For this review, take the finished solid that the model builds, in its own axes (mm). Face numbers are marked on the shaded views. A direction names the side the tool comes from. Round coordinates to 2 decimals unless told otherwise and drop trailing zeros. Order: outer loops, then holes, each group sorted by start corner. A loop starts at its lowest first (then second) coordinate and runs counter-clockwise, first axis right, second up.
from build123d import *

# Parameters (mm, degrees)
F0_W      = 143.89868
F0_H      = 139.25679
F1_DEPTH  = 152.4
F2_W      = 25.4
F2_H      = 25.4
F2_W_2    = 35.657714
F2_H_2    = 78.153904
F3_DEPTH  = 142.24
F4_W      = 129.092633
F4_H      = 89.404348
F5_DEPTH  = 50.8
F6_W      = 134.386524
F6_H      = 100.197379
F7_DEPTH  = 50.8
F8_W      = 129.092633
F8_H      = 8.289584
F9_DEPTH  = 50.8
F10_W     = 25.4
F10_H     = 25.4
F11_DEPTH = 25.4
F12_W     = 25.4
F12_H     = 25.4
F13_DEPTH = 50.8
F14_W     = 25.399997
F14_H     = 25.4
F14_W_2   = 25.4
F15_DEPTH = 25.4


with BuildPart() as f1:
    # F0 (on Front) → F1 (new body)
    with BuildSketch(Plane.XZ):
        Rectangle(F0_W, F0_H)
    extrude(amount=F1_DEPTH)

    # F2 (on face) → F3 (cut)
    with BuildSketch(Plane.XZ.offset(152.4)):
        with Locations((-40.786578, 12.7)):
            Rectangle(F2_W, F2_H)
        with Locations((40.542332, 12.7)):
            Rectangle(F2_W, F2_H)
        with Locations((0, -15.630781)):
            Rectangle(F2_W_2, F2_H_2)
    extrude(amount=-F3_DEPTH, mode=Mode.SUBTRACT)

    # F4 (on face) → F5 (cut)
    with BuildSketch(Plane.YZ.offset(-17.828857)):
        with Locations((-79.17279, -1.715975)):
            Rectangle(F4_W, F4_H)
    extrude(amount=-F5_DEPTH, mode=Mode.SUBTRACT)

    # F6 (on face) → F7 (cut)
    with BuildSketch(Plane(origin=(17.828857, 0, 0), x_dir=(0, -1, 0), z_dir=(-1, 0, 0))):
        with Locations((77.042945, -4.609043)):
            Rectangle(F6_W, F6_H)
    extrude(amount=-F7_DEPTH, mode=Mode.SUBTRACT)

    # F8 (on face) → F9 (cut)
    with BuildSketch(Plane.YZ.offset(-17.828857)):
        with Locations((-79.17279, -50.562941)):
            Rectangle(F8_W, F8_H)
    extrude(amount=-F9_DEPTH, mode=Mode.SUBTRACT)

    # F10 (on face) → F11 (cut)
    with BuildSketch(Plane.YZ.offset(71.94934)):
        with Locations((-115.364381, 20.59305)):
            Rectangle(F10_W, F10_H)
        with Locations((-39.158143, 20.59305)):
            Rectangle(F10_W, F10_H)
    extrude(amount=-F11_DEPTH, mode=Mode.SUBTRACT)

    # F12 (on face) → F13 (cut)
    with BuildSketch(Plane(origin=(-71.94934, 0, 0), x_dir=(0, -1, 0), z_dir=(-1, 0, 0))):
        with Locations((46.475742, 16.083911)):
            Rectangle(F12_W, F12_H)
        with Locations((105.357133, 16.083911)):
            Rectangle(F12_W, F12_H)
    extrude(amount=-F13_DEPTH, mode=Mode.SUBTRACT)

    # F14 (on face) → F15 (cut)
    with BuildSketch(Plane(origin=(0, 0, 0), x_dir=(-1, 0, 0), z_dir=(0, 1, 0))):
        with Locations((-26.893279, 13.194072)):
            Rectangle(F14_W, F14_H)
        with Locations((27.382654, 13.194072)):
            Rectangle(F14_W_2, F14_H)
    extrude(amount=-F15_DEPTH, mode=Mode.SUBTRACT)


solid = f1.part
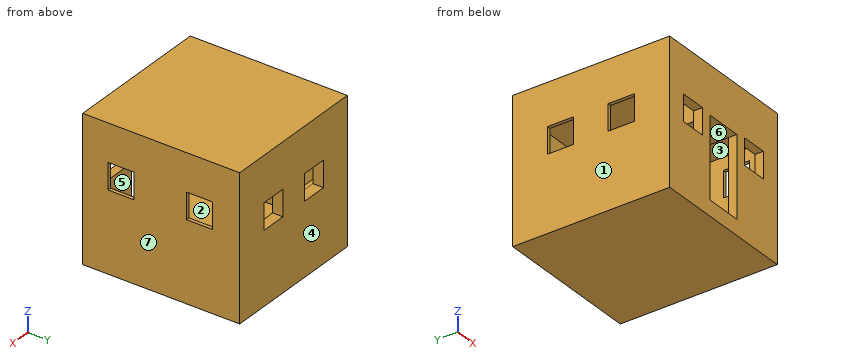
(1) Add section B-B on z = -31. Give the boundary of the cut face in (x, y).
(2) Add section D-D on y = -70. Give the boundary of the cut face in (x, z).
(3) Add section C-C on x = -4. Give the boundary of the cut face in (y, z), plus the area to 3 significant figures.
(4) Tool access review of the marked faces 5, 6 and 7: name each direction out of +Z, -Z, +X, -X, +Y, -Y from which nothing blocks a thin tool from reaching the whole face with its end or side.
(5) Draft analysis for pull direction X (two halves, no side actions). For the marked faces 1, 2, 3 and 4, state which applies: pulls with the +X half, pulls with the -X half, needs draft (parallel to the pull), parting line crosses it, or undercut.
(6) Add section A-A on y = -105.5. Give the boundary of the cut face in (x, z).
(7) Clearance check with flat-ended pins moving along their axes: P1, Ø12, axis at x = -14, z = -10.5, coming from the -Y side; P2, Ø2.5, axis at x = 16.5, z = 24.5, coming from the +Y side. State where each tip first meets the part, or that it passes through.
(8) Wall thickness on L1, parallel to X at y = -75, z = 35.5; L2, parallel to Z at x = 37.5, y = -63; L3, parallel to X at y = -118.5, z = -29: over which ranges is each line inside the solid? List them lowest first.
Here are the results:
1. outline: (-71.95, -152.4) - (-17.83, -152.4) - (-17.83, -143.72) - (-68.63, -143.72) - (-68.63, -14.63) - (-17.83, -14.63) - (-17.83, -10.16) - (17.83, -10.16) - (17.83, -9.85) - (68.63, -9.85) - (68.63, -144.24) - (17.83, -144.24) - (17.83, -152.4) - (71.95, -152.4) - (71.95, 0) - (-71.95, 0) - close
2. outline: (-71.95, -69.63) - (71.95, -69.63) - (71.95, 69.63) - (-71.95, 69.63) - close; hole (-68.63, -54.71) - (68.63, -54.71) - (68.63, 45.49) - (17.83, 45.49) - (17.83, 23.45) - (-17.83, 23.45) - (-17.83, 42.99) - (-68.63, 42.99) - close
3. outline: (-152.4, -69.63) - (0, -69.63) - (0, 69.63) - (-152.4, 69.63) - (-152.4, 23.45) - (-10.16, 23.45) - (-10.16, -54.71) - (-152.4, -54.71) - close
3. area: 10,100 mm2
4. face 5: none
4. face 6: -Y
4. face 7: +Z, -Z, +X, +Y, -Y
5. face 1: pulls with the -X half
5. face 2: undercut
5. face 3: undercut
5. face 4: needs draft
6. outline: (-71.95, -69.63) - (71.95, -69.63) - (71.95, 7.89) - (68.63, 7.89) - (68.63, -54.71) - (-68.63, -54.71) - (-68.63, 3.38) - (-71.95, 3.38) - close; (-71.95, 28.78) - (-68.63, 28.78) - (-68.63, 42.99) - (-17.83, 42.99) - (-17.83, 23.45) - (17.83, 23.45) - (17.83, 45.49) - (68.63, 45.49) - (68.63, 33.29) - (71.95, 33.29) - (71.95, 69.63) - (-71.95, 69.63) - close
7. P1: stops at y = -152.4
7. P2: stops at y = -25.4
8. L1: x = -71.95 to -68.63, -17.83 to 17.83, 68.63 to 71.95
8. L2: z = -69.63 to -54.71, 45.49 to 69.63
8. L3: x = -71.95 to -68.63, 68.63 to 71.95
